Part model, mm, in its own coordinate system. A direction names the side the tool comes from. Give positions to 0.01 mm unless a question says otherwise; leave off trailing zeros. Order: outer loops, then holes, each group sorted by start corner. A loop starts at its lowest first (then second) coordinate and runs counter-clockwise, first axis right, second up. Notation, with made-up numbers: (-10.75, 28.5) - (4.25, 28.5) arc R26 ccw to (4.25, 55.5) - close; hole circle Ø9 at (34, -1). An arc over 180 degrees is marked (long way). One line per item, written item: value.
```python
from build123d import *

# Parameters (mm, degrees)
SKETCH2_R           = 13.5
BOSS_EXTRUDE1_DEPTH = 32
SKETCH4_R           = 11
CUT_EXTRUDE1_DEPTH  = 10
SKETCH5_R           = 7.5
CUT_EXTRUDE2_DEPTH  = 30


with BuildPart() as part:
    # Sketch2 → Boss-Extrude1 (new body)
    with BuildSketch(Plane.XY):
        Circle(SKETCH2_R)
    extrude(amount=-BOSS_EXTRUDE1_DEPTH)

    # Sketch4 → Cut-Extrude1 (cut)
    with BuildSketch(Plane.XY):
        Circle(SKETCH4_R)
    extrude(amount=-CUT_EXTRUDE1_DEPTH, mode=Mode.SUBTRACT)

    # Sketch5 → Cut-Extrude2 (cut)
    with BuildSketch(Plane.XY):
        Circle(SKETCH5_R)
    extrude(amount=-CUT_EXTRUDE2_DEPTH, mode=Mode.SUBTRACT)


solid = part.part
```
1) Drill centre lines: line 1 along Y through (x, z) = (0, -1.75); line 2 along Y through (x, z) = (0, -20.75); line 3 along Z through (x, y) = (7.5, -7.25). Where is each one in solid material? Low to high. Write a range as from..to.
Outcome:
line 1: y = -13.5..-11, 11..13.5
line 2: y = -13.5..-7.5, 7.5..13.5
line 3: z = -32..-10
2) Cut at D-D, the plane y = -9.5. Give the cut face in (x, z).
Outcome:
outline: (-9.59, -32) - (9.59, -32) - (9.59, 0) - (5.55, 0) - (5.55, -10) - (-5.55, -10) - (-5.55, 0) - (-9.59, 0) - close
3) Mould opens along X. For faces 1 (the cylindrical face through (-2.93, -13.18, -15.78)), 2 (the cylindrical face through (-7.493, 0.33, -19.86)), 3 (the flat face through (-5, -10, 0)) say: released by +X, released by -X, zero draft, split by the parting line, or undercut.
Outcome:
face 1: split by the parting line
face 2: undercut
face 3: zero draft
4) Cut at A-A, the plane y = 0. Give the cut face in (x, z), then the cut area to 3 significant figures.
Outcome:
outline: (-13.5, -32) - (13.5, -32) - (13.5, 0) - (11, 0) - (11, -10) - (7.5, -10) - (7.5, -30) - (-7.5, -30) - (-7.5, -10) - (-11, -10) - (-11, 0) - (-13.5, 0) - close
area: 344 mm^2
5) Which spindle directions (+Z, -Z, +X, -X, +Y, -Y) get a long thin tool onto all of the face, cutting with end or side? Do faces 4 (the cylindrical face through (-2.38, -10.74, -4.93)), 5 (the flat face through (0, 0, -32)). Say none if no direction does.
Outcome:
face 4: +Z
face 5: -Z, +X, -X, +Y, -Y
6) Pin check, flat tips, straight feed: pin 1 (1 mm diameter, centred on x = -7, y = 8, fed in from +Z); pin 2 (12 mm diameter, centred on x = 1, y = 0.5, fed in from +Z); pin 3 (3 mm diameter, centred on y = -3, z = -26.5, fed in from +X); pin 4 (1 mm diameter, centred on x = 5, y = 9, fed in from +Z). Stop position of each tip, or through.
Outcome:
pin 1: stops at z = 0
pin 2: stops at z = -30
pin 3: stops at x = 13.42
pin 4: stops at z = -10
7) Cut at B-B, the plane z = -19.5. Give the cut face in (x, y).
Outcome:
outline: circle Ø27 at (0, 0); hole circle Ø15 at (0, 0)
